from build123d import *

# Parameters (mm, degrees)
ESQUISSE1_R             = 1.15
BOSS_EXTRU_1_DEPTH      = 1.8
BOSS_EXTRU_2_DEPTH      = 8
ENL_V_MAT_EXTRU_1_DEPTH = 7
ESQUISSE4_W             = 3.5
ESQUISSE4_H             = 0.873592076
ENL_V_MAT_EXTRU_2_DEPTH = 1
ESQUISSE5_W             = 1
ESQUISSE5_H             = 1
ENL_V_MAT_EXTRU_3_DEPTH = 11
ESQUISSE6_W             = 6.2
ESQUISSE6_H             = 3.3
ENL_V_MAT_EXTRU_4_DEPTH = 1
CHANFREIN1_SIZE         = 1
ESQUISSE7_R             = 6
BOSS_EXTRU_3_DEPTH      = 6.8
CONG_1_R                = 0.5
ESQUISSE8_R             = 1.3
ENL_V_MAT_EXTRU_5_DEPTH = 2


with BuildPart() as part:
    # Esquisse1 → Boss.-Extru.1 (new body)
    with BuildSketch(Plane.XY):
        with BuildLine():
            Line((-12.744645331, 10.992907801), (-4.994645331, 10.992907801))
            ThreePointArc((-4.994645331, 10.992907801), (-2.744645331, 8.742907801), (-0.494645331, 10.992907801))
            Line((-0.494645331, 10.992907801), (7.255354669, 10.992907801))
            Line((7.255354669, 10.992907801), (7.255354669, 3.192907801))
            ThreePointArc((7.255354669, 3.192907801), (9.455354669, 0.992907801), (7.255354669, -1.207092199))
            Line((7.255354669, -1.207092199), (7.255354669, -9.007092199))
            Line((7.255354669, -9.007092199), (-0.494645331, -9.007092199))
            ThreePointArc((-0.494645331, -9.007092199), (-2.744645331, -6.757092199), (-4.994645331, -9.007092199))
            Line((-4.994645331, -9.007092199), (-12.744645331, -9.007092199))
            Line((-12.744645331, -9.007092199), (-12.744645331, -1.207092199))
            ThreePointArc((-12.744645331, -1.207092199), (-14.944645331, 0.992907801), (-12.744645331, 3.192907801))
            Line((-12.744645331, 3.192907801), (-12.744645331, 10.992907801))
        make_face()
        with Locations((-12.744645331, 0.992907801)):
            Circle(ESQUISSE1_R, mode=Mode.SUBTRACT)
        with Locations((7.255354669, 0.992907801)):
            Circle(ESQUISSE1_R, mode=Mode.SUBTRACT)
    extrude(amount=BOSS_EXTRU_1_DEPTH)

    # Esquisse2 → Boss.-Extru.2 (add)
    with BuildSketch(Plane.XY.offset(1.8)):
        Polygon((-8.744645331, -7.507092199), (3.255354669, -7.507092199), (3.255354669, -6.707092199), (2.255354669, -6.707092199), (2.255354669, -4.407092199), (3.255354669, -4.407092199), (3.255354669, -2.507092199), (-8.744645331, -2.507092199), (-8.744645331, -4.407092199), (-7.744645331, -4.407092199), (-7.744645331, -6.707092199), (-8.744645331, -6.707092199), align=None)
    extrude(amount=BOSS_EXTRU_2_DEPTH)

    # Esquisse3 → Enlèv. mat.-Extru.1 (cut)
    with BuildSketch(Plane.XY.offset(9.8)):
        Polygon((-6.444645331, -3.707092199), (0.955354669, -3.707092199), (0.955354669, -2.907092199), (1.755354669, -2.907092199), (1.755354669, -3.707092199), (1.755354669, -6.707092199), (-7.244645331, -6.707092199), (-7.244645331, -3.707092199), (-7.244645331, -2.907092199), (-6.444645331, -2.907092199), align=None)
    extrude(amount=-ENL_V_MAT_EXTRU_1_DEPTH, mode=Mode.SUBTRACT)

    # Esquisse4 → Enlèv. mat.-Extru.2 (cut)
    with BuildSketch(Plane(origin=(0, -2.507092199, 0), x_dir=(1, 0, 0), z_dir=(0, 1, 0))):
        Polygon((-8.744645331, -1.8), (3.255354669, -1.8), (3.255354669, -2.8), (0.455354669, -2.8), (0.455354669, -9.8), (-5.944645331, -9.8), (-5.944645331, -2.8), (-8.744645331, -2.8), align=None)
        with Locations((-2.744645331, -6.063203962)):
            Rectangle(ESQUISSE4_W, ESQUISSE4_H, mode=Mode.SUBTRACT)
    extrude(amount=-ENL_V_MAT_EXTRU_2_DEPTH, mode=Mode.SUBTRACT)

    # Esquisse5 → Enlèv. mat.-Extru.3 (cut)
    with BuildSketch(Plane(origin=(0, -2.507092199, 0), x_dir=(1, 0, 0), z_dir=(0, 1, 0))):
        with Locations((-8.244645331, -9.3)):
            Rectangle(ESQUISSE5_W, ESQUISSE5_H)
        with Locations((2.755354669, -9.3)):
            Rectangle(ESQUISSE5_W, ESQUISSE5_H)
    extrude(amount=-ENL_V_MAT_EXTRU_3_DEPTH, mode=Mode.SUBTRACT)

    # Esquisse6 → Enlèv. mat.-Extru.4 (cut)
    with BuildSketch(Plane(origin=(0, -3.507092199, 0), x_dir=(1, 0, 0), z_dir=(0, 1, 0))):
        with Locations((-2.744645331, -8.15)):
            Rectangle(ESQUISSE6_W, ESQUISSE6_H)
    extrude(amount=-ENL_V_MAT_EXTRU_4_DEPTH, mode=Mode.SUBTRACT)

    # Chanfrein1
    # the kernel refuses this chamfer: 1 mm, written as the material it takes off along each edge
    with BuildSketch(Plane(origin=(1.577037657, -2.507092199, 6.5), x_dir=(0, -0.9996219169112968, 0.027495876610586487), z_dir=(-1, 0, 0))) as chanfrein1_piece_1_section:
        Polygon((CHANFREIN1_SIZE * 0.999621916911, -CHANFREIN1_SIZE * 0.0274958766106), (-CHANFREIN1_SIZE * 0.0274958766106, -CHANFREIN1_SIZE * 0.999621916911), (0, 0), align=None)
    chanfrein1_piece_1 = extrude(amount=6.071682988, mode=Mode.PRIVATE)
    chanfrein1_piece_1 = split(chanfrein1_piece_1, bisect_by=Plane(origin=(0.455354669, -3.107092199, 6.3), z_dir=(-1, 0, 0)), keep=Keep.TOP, mode=Mode.PRIVATE)
    add(chanfrein1_piece_1, mode=Mode.SUBTRACT)

    # Esquisse7 → Boss.-Extru.3 (add)
    with BuildSketch(Plane.XY.offset(1.8)):
        with Locations(Location((-2.744645331, 4.992907801, 0), (0, 0, 111.61384575))):
            Circle(ESQUISSE7_R)
    extrude(amount=BOSS_EXTRU_3_DEPTH)

    # Congé1
    cong_1_edges = [part.edges().sort_by_distance(p)[0] for p in [
        (-0.534549974, -0.585217199, 8.6),
    ]]
    fillet(cong_1_edges, radius=CONG_1_R)

    # Esquisse8 → Enlèv. mat.-Extru.5 (cut)
    with BuildSketch(Plane.XY.offset(8.6)):
        with Locations((-2.744645331, 4.992907801)):
            Circle(ESQUISSE8_R)
    extrude(amount=-ENL_V_MAT_EXTRU_5_DEPTH, mode=Mode.SUBTRACT)


solid = part.part
Build history of the part. All positions in model axes, mm. A direction names the side the tool comes from. Coordinates: 2 decimals unless noted, no trailing zeros. Order: outer loops, then holes, each group sorted by start corner. A loop starts at its lowest first (then second) coordinate and runs counter-clockwise, first axis right, second up. Notation, with made-up numbers: (-29.5, -36) -> (24.5, -36) arc R7 ccw to (24.5, -30) -> close; hole circle Ø2 at (65.25, -7). An arc over 180 degrees is marked (long way). One line per item, written item: value.
(1) Slice it at B-B, the plane x = 8. List the corners of the cut face in (y, z).
Checked values:
outline: (-1.08, 0) -> (0.12, 0) -> (0.12, 1.8) -> (-1.08, 1.8) -> close; (1.87, 0) -> (3.06, 0) -> (3.06, 1.8) -> (1.87, 1.8) -> close
(2) Slice it at C-C, the plane z = 2.25. List the corners of the cut face in (x, y), plus the area to 3 significant figures.
Checked values:
outline: (-8.74, -7.51) -> (3.26, -7.51) -> (3.26, -6.71) -> (2.26, -6.71) -> (2.26, -4.41) -> (3.26, -4.41) -> (3.26, -3.51) -> (-8.74, -3.51) -> (-8.74, -4.41) -> (-7.74, -4.41) -> (-7.74, -6.71) -> (-8.74, -6.71) -> close; circle Ø12 at (-2.74, 4.99)
area: 156 mm2
(3) Slice it at D-D, the plane y = -1.5. List the corners of the cut face in (x, z), plus the area to 3 significant figures.
Checked values:
outline: (-12.74, 0) -> (7.26, 0) -> (7.26, 1.8) -> (-12.74, 1.8) -> close
area: 36.0 mm2
(4) Probe line 1 (X direction, y = -5, z = 3.5); line 2 (Z direction, x = -6.5, y = 5); line 3 (X direction, y = -7, z = 1.5). List the from-to ranges inside material, lowest first. Write a range as [from, to].
Checked values:
line 1: [-7.74, -7.24], [1.76, 2.26]
line 2: [0, 8.6]
line 3: [-12.74, -3.76], [-1.73, 7.26]
(5) Drop flat-ended pins along their axis: pin 1 Ø3 at (x, y) = (-12.74, 0.99) entering from +Z; pin 2 Ø6 at (x, y) = (4, 5) entering from +Z; pin 3 Ø4 at (x, z) = (6.5, 5.5) entering from -Y; pin 4 Ø0.5 at (x, z) = (-8, 6.5) entering from -Y. Give the stop position or say it passes through.
Checked values:
pin 1: z = 1.8
pin 2: z = 8.6
pin 3: through
pin 4: y = -7.51
(6) Slice it at A-A, the plane z = 7. Count the separate pieces of the cut face and the enclosed holes in it, plus the area to 3 significant figures.
Checked values:
separate pieces: 2
enclosed holes: 1
area: 127 mm2
(7) Mould opens along Z. For faces 4 (the flat face through (-3, 1, 0)), 5 (the flat face through (-4.495, -3.3, 5.9)), 6 (the flat face through (-3, -3.507, 4)) say: pulls with the +Z half, pulls with the -Z half, needs draft (parallel to the pull), parting line crosses it, or undercut.
Checked values:
face 4: pulls with the -Z half
face 5: needs draft
face 6: undercut
(8) Tool access for faces 1 (the flat face through (-3, -3, 5.626)), 2 (the flat face through (-3, 10, 1.8)), 3 (the flat face through (7.255, -5, 1)): list every direction of +Z, -Z, +X, -X, +Y, -Y with a clear straight run to the whole face (end or side of a thin tool).
Checked values:
face 1: none
face 2: -Z, +Y
face 3: +Z, -Z, +X, -Y
